Read the model definition and answer for the solid it produces. Units are mm, in the model's axes. Coordinates: 2 decimals unless noted, no trailing zeros. Write each loop counter-clockwise with the first axis right and the second up, starting at its lowest first coordinate (ties: lowest second). Pieces come first, ordered by that corner, then holes.
1) The part is cut by section B-B (z = -1.75). Determine the outline of the cut face in (x, y), then the cut area to 3 significant figures.
2) Determine the mould class of faces 1 (the face through (-3, 0, 0)), 2 (the face through (0, -4, 4)), 3 (the face through (-2.17, -9.76, -3.58)) for opening direction Y: +Y half, -Y half, draft (parallel to the pull), parting line (faces both ways), or undercut.
3) Find the intervals of material crossed by line 1 (Y direction, x = 0, z = -2); line 2 (Y direction, x = -1.5, z = -0.75); line 3 (X direction, y = 1.5, z = 2.25), in increasing order.
4) The part is cut by section A-A (z = 3). Determine the outline of the cut face in (x, y), then the cut area to 3 significant figures.
5) Each of these flat-tipped pins is pushed along its axis until it touches: pin 1 Ø2 at (x, z) = (-3, 1.5) entering from +Y; pin 2 Ø4 at (x, z) = (3, -1) entering from -Y; pin 3 Ø1 at (y, z) = (-5.5, 3) entering from -X. Where does it stop, or does it pass through?
from build123d import *

# Parameters (mm, degrees)
F2_SIZE = 0.1


# Not quite as in the source:
# - a fillet or chamfer that OpenCascade refuses, or shapes differently, is made with other operations: its cross-section is extruded or revolved along the edge and cut away or added


with BuildPart() as f1:
    # F0 (on Front) → F1 (revolve)
    with BuildSketch(Plane.XZ):
        with BuildLine():
            Line((10, 4), (3, 4))
            Line((3, 4), (3, 0))
            Line((3, 0), (3, -4))
            Line((3, -4), (10, -4))
            Line((10, -4), (10, -3.2615188186))
            ThreePointArc((10, -3.2615188186), (9.9141508898, -2.6119993954), (9.6624996151, -2.0070885037))
            ThreePointArc((9.6624996151, -2.0070885037), (9.2598575755, -1.0392310772), (9.1224989992, 0))
            ThreePointArc((9.1224989992, 0), (9.2598575755, 1.0392310772), (9.6624996151, 2.0070885037))
            ThreePointArc((9.6624996151, 2.0070885037), (9.9141508898, 2.6119993954), (10, 3.2615188186))
            Line((10, 3.2615188186), (10, 4))
        make_face()
    revolve(axis=Axis((0, 0, 5.2388195913), (0, 0, 1)))

    # F2
    f2_edges = [f1.edges().sort_by_distance(p)[0] for p in [
        (-10, 0, 4),
        (-10, 0, -4),
    ]]
    chamfer(f2_edges, length=F2_SIZE)

    # F3: chamfer of 0.5 on 3 edges, made by hand

    # F3_s1 → F3_t2 (revolve, cut)
    with BuildSketch(Plane.XZ):
        Polygon((3.5, 4), (3, 3.5), (3, 4), align=None)
    revolve(axis=Axis((0, 0, 4), (0, 0, 1)), mode=Mode.SUBTRACT)

    # F3_s3 → F3_t4 (revolve, cut)
    with BuildSketch(Plane.XZ):
        Polygon((3, -3.5), (3.5, -4), (3, -4), align=None)
    revolve(axis=Axis((0, 0, -4), (0, 0, 1)), mode=Mode.SUBTRACT)

    # F3_s5 → F3_t6 (revolve, cut)
    with BuildSketch(Plane.XZ):
        Polygon((10.0464466094, 3.8535533906), (9.6928932188, 4), (9.9, 4), align=None)
    revolve(axis=Axis((0, 0, 4), (0, 0, 1)), mode=Mode.SUBTRACT)


solid = f1.part
Reported:
1. outline: circle Ø19.05 at (0, 0); hole circle Ø6 at (0, 0)
1. area: 257 mm2
2. face 1: undercut
2. face 2: draft
2. face 3: parting line
3. line 1: y = -9.66 to -3, 3 to 9.66
3. line 2: y = -9.07 to -2.6, 2.6 to 9.07
3. line 3: x = -9.67 to -2.6, 2.6 to 9.67
4. outline: circle Ø19.97 at (0, 0); hole circle Ø6 at (0, 0)
4. area: 285 mm2
5. pin 1: stops at y = 9.51
5. pin 2: stops at y = -9.75
5. pin 3: stops at x = -8.65
